Part model, mm, in its own coordinate system. Face numbers are marked on the shaded views. A direction names the side the tool comes from. Round coordinates to 2 decimals unless told otherwise and drop trailing zeros. Loops run counter-clockwise (first coordinate to the right, second up) from the corner with the lowest first, then second, coordinate; pieces in that order, holes last. Notation, with made-up numbers: (-7.5, 20) - (23.5, 20) arc R13 ccw to (23.5, 32) - close; hole circle Ø8 at (-26.75, 75). An arc over 180 degrees is marked (long way). Put each result on its own line as item: value.
from build123d import *

# Parameters (mm, degrees)
F0_R      = 37.5
F0_R_2    = 1
F0_R_3    = 3
F1_DEPTH  = 3
F2_R      = 8
F2_R_2    = 3
F3_DEPTH  = 5
F4_SIZE2  = 4.99999
F4_SIZE   = 1.99999
F5_SIZE   = 1
F7_DEPTH  = 8.001
F8_R      = 1.5
F9_DEPTH  = 3.001
F10_W     = 26.2
F10_H     = 22.5
F11_DEPTH = 9
F12_W     = 22.6
F12_H     = 18.9
F13_DEPTH = 4
F14_R     = 3.99999
F15_W     = 4
F15_H     = 22.5
F16_DEPTH = 9
F18_DEPTH = 25


# Not quite as in the source:
# - a fillet or chamfer is up to 0.001 mm smaller than in the source, because OpenCascade refuses the exact size


with BuildPart() as f1:
    # F0 (on Top) → F1 (new body)
    with BuildSketch(Plane.XY):
        Circle(F0_R)
        with Locations((0, -33.5)):
            Circle(F0_R_2, mode=Mode.SUBTRACT)
        with Locations((-33.5, 0)):
            Circle(F0_R_2, mode=Mode.SUBTRACT)
        Circle(F0_R_3, mode=Mode.SUBTRACT)
        with Locations((33.5, 0)):
            Circle(F0_R_2, mode=Mode.SUBTRACT)
        with Locations((0, 33.5)):
            Circle(F0_R_2, mode=Mode.SUBTRACT)
    extrude(amount=F1_DEPTH)

    # F2 (on face) → F3 (join)
    with BuildSketch(Plane.XY.offset(3)):
        Circle(F2_R)
        Circle(F2_R_2, mode=Mode.SUBTRACT)
    extrude(amount=F3_DEPTH)

    # F4 (size 2 and 5 in the source; OpenCascade refuses exactly that, so slightly less here)
    f4_edges = [f1.edges().sort_by_distance(p)[0] for p in [
        (-8, 0, 8),
    ]]
    f4_side = f1.faces().sort_by_distance((-7.773726, 0, 8))[0]
    chamfer(f4_edges, length=F4_SIZE, length2=F4_SIZE2, reference=f4_side)

    # F5
    f5_edges = [f1.edges().sort_by_distance(p)[0] for p in [
        (-3, 0, 0),
        (3, 0, 4),
        (-3, 0, 8),
    ]]
    chamfer(f5_edges, length=F5_SIZE)

    # F6 (on face) → F7 (cut, through all)
    with BuildSketch(Plane(origin=(0, 0, 0), x_dir=(1, 0, 0), z_dir=(0, 0, -1))):
        with BuildLine():
            Line((-1.7286498598, 1.8739716279), (-2.9167940342, 2.7372089))
            ThreePointArc((-2.9167940342, 2.7372089), (-3.2360679775, 2.3511410092), (-3.5045792865, 1.9281919056))
            Line((-3.5045792865, 1.9281919056), (-2.3164351121, 1.0649546335))
            Line((-2.3164351121, 1.0649546335), (-1.7286498598, 1.8739716279))
        make_face()
        with BuildLine():
            Line((1.2480707441, 2.2231327936), (1.7019014352, 3.6198800401))
            ThreePointArc((1.7019014352, 3.6198800401), (1.2360679775, 3.8042260652), (0.7508449189, 3.9288970345))
            Line((0.7508449189, 3.9288970345), (0.2970142278, 2.5321497879))
            Line((0.2970142278, 2.5321497879), (1.2480707441, 2.2231327936))
        make_face()
        with BuildLine():
            ThreePointArc((0.7508449189, 3.9288970345), (1.2360679775, 3.8042260652), (1.7019014352, 3.6198800401))
            Line((1.7019014352, 3.6198800401), (3.1021727103, 7.9294718913))
            Line((3.1021727103, 7.9294718913), (2.151116194, 8.2384888857))
            Line((2.151116194, 8.2384888857), (0.7508449189, 3.9288970345))
        make_face()
        with BuildLine():
            Line((8.5, -0.5), (8.5, 0.5))
            Line((8.5, 0.5), (3.9686269666, 0.5))
            ThreePointArc((3.9686269666, 0.5), (3.9921490369, 0.2504916502), (4, 0))
            ThreePointArc((4, 0), (3.9921490369, -0.2504916502), (3.9686269666, -0.5))
            Line((3.9686269666, -0.5), (8.5, -0.5))
        make_face()
        with BuildLine():
            Line((3.1021727103, -7.9294718913), (1.7019014352, -3.6198800401))
            ThreePointArc((1.7019014352, -3.6198800401), (1.2360679775, -3.8042260652), (0.7508449189, -3.9288970345))
            Line((0.7508449189, -3.9288970345), (2.151116194, -8.2384888857))
            Line((2.151116194, -8.2384888857), (3.1021727103, -7.9294718913))
        make_face()
        with BuildLine():
            ThreePointArc((4, 0), (3.9921490369, 0.2504916502), (3.9686269666, 0.5))
            Line((3.9686269666, 0.5), (2.5, 0.5))
            Line((2.5, 0.5), (2.5, -0.5))
            Line((2.5, -0.5), (3.9686269666, -0.5))
            ThreePointArc((3.9686269666, -0.5), (3.9921490369, -0.2504916502), (4, 0))
        make_face()
        with BuildLine():
            ThreePointArc((0.7508449189, -3.9288970345), (1.2360679775, -3.8042260652), (1.7019014352, -3.6198800401))
            Line((1.7019014352, -3.6198800401), (1.2480707441, -2.2231327936))
            Line((1.2480707441, -2.2231327936), (0.2970142278, -2.5321497879))
            Line((0.2970142278, -2.5321497879), (0.7508449189, -3.9288970345))
        make_face()
        with BuildLine():
            Line((-6.582751826, -5.4006831417), (-2.9167940342, -2.7372089))
            ThreePointArc((-2.9167940342, -2.7372089), (-3.2360679775, -2.3511410092), (-3.5045792865, -1.9281919056))
            Line((-3.5045792865, -1.9281919056), (-7.1705370783, -4.5916661473))
            Line((-7.1705370783, -4.5916661473), (-6.582751826, -5.4006831417))
        make_face()
        with BuildLine():
            ThreePointArc((-3.5045792865, -1.9281919056), (-3.2360679775, -2.3511410092), (-2.9167940342, -2.7372089))
            Line((-2.9167940342, -2.7372089), (-1.7286498598, -1.8739716279))
            Line((-1.7286498598, -1.8739716279), (-2.3164351121, -1.0649546335))
            Line((-2.3164351121, -1.0649546335), (-3.5045792865, -1.9281919056))
        make_face()
        with BuildLine():
            ThreePointArc((-3.5045792865, 1.9281919056), (-3.2360679775, 2.3511410092), (-2.9167940342, 2.7372089))
            Line((-2.9167940342, 2.7372089), (-6.582751826, 5.4006831417))
            Line((-6.582751826, 5.4006831417), (-7.1705370783, 4.5916661473))
            Line((-7.1705370783, 4.5916661473), (-3.5045792865, 1.9281919056))
        make_face()
    extrude(amount=-F7_DEPTH, mode=Mode.SUBTRACT)

    # F8 (on face) → F9 (cut, through all)
    with BuildSketch(Plane.XY.offset(3)):
        with Locations((-19.1, 3)):
            Circle(F8_R)
        with Locations((-19.1, -3)):
            Circle(F8_R)
    extrude(amount=-F9_DEPTH, mode=Mode.SUBTRACT)

    # F10 (on face) → F11 (join)
    with BuildSketch(Plane.XY.offset(3)):
        with Locations((-19.1, 0)):
            Rectangle(F10_W, F10_H)
    extrude(amount=F11_DEPTH)

    # F12 (on face) → F13 (cut)
    with BuildSketch(Plane.XY.offset(12)):
        with Locations((-19.1, 0)):
            Rectangle(F12_W, F12_H)
    extrude(amount=-F13_DEPTH, mode=Mode.SUBTRACT)

    # F14 (radius 4 in the source; OpenCascade refuses exactly that, so slightly less here)
    f14_edges = [f1.edges().sort_by_distance(p)[0] for p in [
        (-30.4, 0, 8),
        (-7.8, 0, 8),
    ]]
    fillet(f14_edges, radius=F14_R)

    # F15 (on face) → F16 (cut, through all)
    with BuildSketch(Plane.XY.offset(12)):
        with Locations((-19.1, 0)):
            Rectangle(F15_W, F15_H)
    extrude(amount=-F16_DEPTH, mode=Mode.SUBTRACT)

    # F17 (on face) → F18 (cut, symmetric)
    with BuildSketch(Plane.XZ.offset(-9.45)):
        with BuildLine():
            ThreePointArc((-11.9585715715, 12), (-9.8421848073, 15.2194103823), (-9.1, 19))
            ThreePointArc((-9.1, 19), (-26.8459666924, 25.3245553203), (-17.1, 9.2020410289))
            Line((-17.1, 9.2020410289), (-17.1, 12))
            Line((-17.1, 12), (-11.9585715715, 12))
        make_face()
        with BuildLine():
            Line((-17.1, 12), (-17.1, 9.2020410289))
            ThreePointArc((-17.1, 9.2020410289), (-14.3199820053, 10.2164114412), (-11.9585715715, 12))
            Line((-11.9585715715, 12), (-17.1, 12))
        make_face()
    extrude(amount=F18_DEPTH, both=True, mode=Mode.SUBTRACT)


solid = f1.part
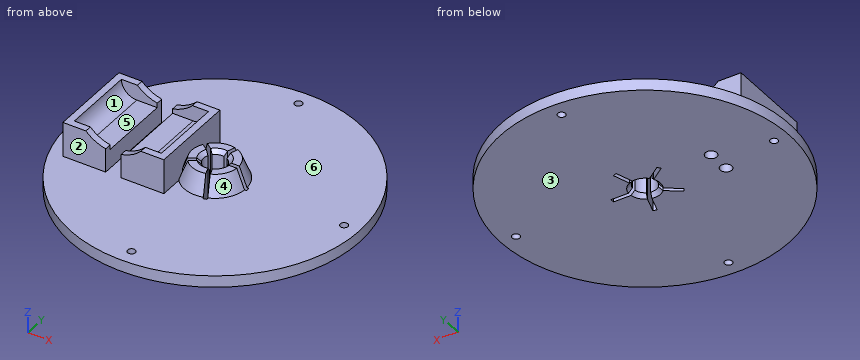
1. Probe line 1 along Y through (x, z) = (-30, 10.75); line 2 along X through (y, z) = (-9, 5); line 3 along Y through (x, z) = (-19.1, 2.1). List the from-to ranges inside material, lowest first. Write a range as [from, to].
A:
line 1: y = [-11.25, -9.45], [9.45, 11.25]
line 2: x = [-32.2, -21.1], [-17.1, -6]
line 3: y = [-32.27, -4.5], [-1.5, 1.5], [4.5, 32.27]
2. Band-saw the part on C-C (x = 14). List the corners of the cut face in (y, z).
A:
outline: (-34.79, 0) - (34.79, 0) - (34.79, 3) - (-34.79, 3) - close
3. Pin check, flat tips, straight feed: P1, Ø1.8, axis at x = -19.1, y = -3, coming from the -Z side; P2, Ø6, axis at x = -9, z = 8.5, coming from the -Y side; P3, Ø1.3, axis at x = 4, y = -4, coming from the +Z side; P4, Ø6, axis at x = 11.5, y = 27, coming from the -Z side. Stop position of each tip, or through.
A:
P1: passes through
P2: stops at y = -11.25
P3: stops at z = 8
P4: stops at z = 0
4. Band-saw the part on A-A (x = 33.5). List the corners of the cut face in (y, z), plus the area to 3 significant figures.
A:
outline: (-16.85, 0) - (-1, 0) - (-1, 3) - (-16.85, 3) - close; (1, 0) - (16.85, 0) - (16.85, 3) - (1, 3) - close
area: 95.1 mm²
5. Band-saw the part on D-D (y = -25). List the corners of the cut face in (x, z).
A:
outline: (-27.95, 0) - (27.95, 0) - (27.95, 3) - (-27.95, 3) - close
6. Tool access for the marked faces 1, 2 and 3: list every direction of +Z, -Z, +X, -X, +Y, -Y with a clear straight run to the whole face (end or side of a thin tool).
A:
face 1: +Z
face 2: +Z, +X, -X, -Y
face 3: -Z, +X, -X, +Y, -Y
7. Two-plate mould, pull along Y, no slides. Class the marked faces 4, 5 and 6: pulls with the +Y half, pulls with the -Y half, needs draft (parallel to the pull), parting line crosses it, or undercut.
A:
face 4: pulls with the -Y half
face 5: undercut
face 6: needs draft
